from build123d import *

# Parameters (mm, degrees)
ESQUISSE1_R                  = 16
ESQUISSE1_R_2                = 2.03
BOSS_EXTRU_1_DEPTH           = 3
ESQUISSE2_R                  = 8
ESQUISSE2_R_2                = 4.02
BOSS_EXTRU_2_DEPTH           = 10
ESQUISSE3_R                  = 4.02
ENL_V_MAT_EXTRU_1_DEPTH      = 27.095976701
ENL_V_MAT_EXTRU_2_DEPTH      = 27.095976701
ENL_V_MAT_EXTRU_2_DEPTH_BACK = 27.095976701
ESQUISSE4_R                  = 1.7


with BuildPart() as part:
    # Esquisse1 → Boss.-Extru.1 (new body)
    with BuildSketch(Plane.XY):
        Circle(ESQUISSE1_R)
        with Locations((-8.407499628, 8.407499628)):
            Circle(ESQUISSE1_R_2, mode=Mode.SUBTRACT)
        with Locations((8.407499628, 8.407499628)):
            Circle(ESQUISSE1_R_2, mode=Mode.SUBTRACT)
        with Locations((8.407499628, -8.407499628)):
            Circle(ESQUISSE1_R_2, mode=Mode.SUBTRACT)
        with Locations((-8.407499628, -8.407499628)):
            Circle(ESQUISSE1_R_2, mode=Mode.SUBTRACT)
    extrude(amount=BOSS_EXTRU_1_DEPTH)

    # Esquisse2 → Boss.-Extru.2 (add)
    with BuildSketch(Plane.XY.offset(3)):
        Circle(ESQUISSE2_R)
        Circle(ESQUISSE2_R_2, mode=Mode.SUBTRACT)
    extrude(amount=BOSS_EXTRU_2_DEPTH)

    # Esquisse3 → Enlèv. mat.-Extru.1 (cut, through all)
    with BuildSketch(Plane.XY.offset(13)):
        Circle(ESQUISSE3_R)
    extrude(amount=-ENL_V_MAT_EXTRU_1_DEPTH, mode=Mode.SUBTRACT)

    # Esquisse4 → Enlèv. mat.-Extru.2 (cut, two sides: drawn at the far end of the back side and taken through both)
    with BuildSketch(Plane(origin=(0, 0, 0), x_dir=(1, 0, 0), z_dir=(0, 1, 0)).offset(-ENL_V_MAT_EXTRU_2_DEPTH_BACK)):
        with Locations(Location((0, -7.8, 0), (0, 0, 270))):
            Circle(ESQUISSE4_R)
    extrude(amount=ENL_V_MAT_EXTRU_2_DEPTH + ENL_V_MAT_EXTRU_2_DEPTH_BACK, mode=Mode.SUBTRACT)


solid = part.part
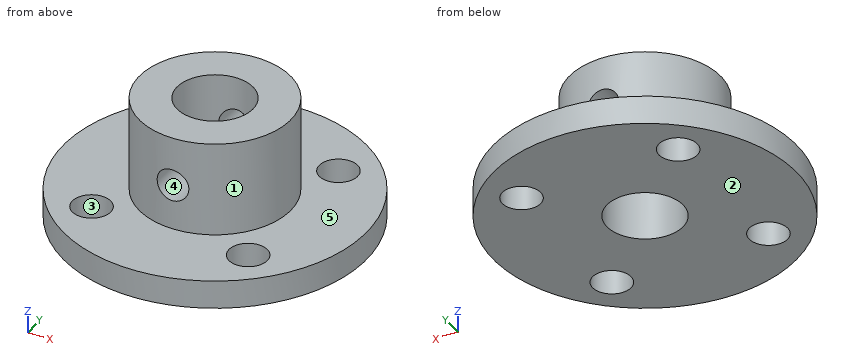
Geometry: final body of the model. Coordinates: model frame, mm. Face numbers are marked on the shaded views. A direction names the side the tool comes from. Coordinates: 2 decimals unless noted, no trailing zeros. Write each loop counter-clockwise with the first axis right and the second up, starting at its lowest first coordinate (ties: lowest second). Pieces come first, ordered by that corner, then holes. Notation, with made-up numbers: (45, 15) - (61, 15) arc R31 ccw to (61, 44) - close; hole circle Ø11 at (-23, 6.25). An arc over 180 degrees is marked (long way). Return JSON: item names as keys, results as strings.
Item 1: Section query D-D (z = 7.8). Output: boundary loops of the cut face in (x, y), and give its area (3 significant figures).
Completed:
{"outline": "(-1.7, -7.82) - (-1.7, -3.64) arc R4.02 cw to (-1.7, 3.64) - (-1.7, 7.82) arc R8 ccw to start; (1.7, -7.82) arc R8 ccw to (1.7, 7.82) - (1.7, 3.64) arc R4.02 cw to (1.7, -3.64) - close", "area": "123 mm2"}
Item 2: Line query: L1, parallel to Z at x = 0, y = 5; L2, parallel to X at y = -9, z = 2.5; L3, parallel to Y at x = 1, z = 12.75. Output: solid intervals per line, ascending.
Completed:
{"L1": "z = 0 to 6.1, 9.5 to 13", "L2": "x = -13.23 to -10.35, -6.47 to 6.47, 10.35 to 13.23", "L3": "y = -7.94 to -3.89, 3.89 to 7.94"}
Item 3: Section query A-A (y = 0). Output: boundary loops of the cut face in (x, z).
Completed:
{"outline": "(-16, 0) - (-4.02, 0) - (-4.02, 13) - (-8, 13) - (-8, 3) - (-16, 3) - close; (4.02, 0) - (16, 0) - (16, 3) - (8, 3) - (8, 13) - (4.02, 13) - close"}
Item 4: Pull-direction query (X, two-part tool) for the marked faces 1, 2 and 3; classes: +X half, -X half, draft (parallel to the pull), parting line (faces both ways), or undercut.
Completed:
{"face 1": "parting line", "face 2": "draft", "face 3": "undercut"}
Item 5: Pin query (flat end, axial travel): pin 1 Ø7 at (x, y) = (0, 0) entering from +Z (3 decimals); pin 2 Ø2 at (x, z) = (5, 9) entering from -Y; pin 3 Ø6 at (x, y) = (-4, -11) entering from +Z; pin 4 Ø2 at (x, z) = (2.5, 1.5) entering from +Y. Return the tip coordinate at first contact, or that it passes through.
Completed:
{"pin 1": "passes through", "pin 2": "stops at y = -6.93", "pin 3": "stops at z = 3", "pin 4": "stops at y = 15.93"}
Item 6: Reachability of the marked faces 4 and 5 from +Z, -Z, +X, -X, +Y, -Y: full face, straight path, thin tool, end or side. Return the list, or none.
Completed:
{"face 4": "+Y, -Y", "face 5": "+Z"}
Item 7: Section query B-B (y = 7.5). Output: boundary loops of the cut face in (x, z).
Completed:
{"outline": "(-14.13, 0) - (-10.22, 0) - (-10.22, 3) - (-14.13, 3) - close; (-6.59, 0) - (6.59, 0) - (6.59, 3) - (2.78, 3) - (2.78, 13) - (-2.78, 13) - (-2.78, 3) - (-6.59, 3) - close; (10.22, 0) - (14.13, 0) - (14.13, 3) - (10.22, 3) - close; hole circle Ø3.4 at (0, 7.8)"}
Item 8: Section query C-C (x = 0). Output: boundary loops of the cut face in (y, z).
Completed:
{"outline": "(-16, 0) - (-4.02, 0) - (-4.02, 6.1) - (-8, 6.1) - (-8, 3) - (-16, 3) - close; (-8, 9.5) - (-4.02, 9.5) - (-4.02, 13) - (-8, 13) - close; (4.02, 0) - (16, 0) - (16, 3) - (8, 3) - (8, 6.1) - (4.02, 6.1) - close; (4.02, 9.5) - (8, 9.5) - (8, 13) - (4.02, 13) - close"}
